For this review, take the finished solid that the model builds, in its own axes (mm). A direction names the side the tool comes from. Give positions to 0.01 mm unless a question says otherwise; leave off trailing zeros. Loops run counter-clockwise (first coordinate to the right, second up) from the corner with the lowest first, then second, coordinate; pieces in that order, holes last. Notation, with made-up numbers: (6, -37.5) -> (10, -37.5) arc R32 ccw to (10, -5.5) -> close; hole circle Ø10 at (33.5, -11). An arc over 180 degrees is marked (long way). One line per question, with ' | ' between items. Start each with the question number.
(1) Consider section A-A (x = -10). Write out the cut boundary in (y, z).
(2) Consider section C-C (x = 63). Write out the cut boundary in (y, z).
(3) Tool access review of faces 4 (the cylindrical face through (26.393, -27.015, 1.521)), 5 (the cylindrical face through (-61.468, -83.668, 1.479)): name each direction out of +Z, -Z, +X, -X, +Y, -Y from which nothing blocks a thin tool from reaching the whole face with its end or side.
(4) Draft analysis for pull direction Y (two halves, no side actions). For faces 1 (the cylindrical face through (-62.168, 39.968, 1.479)), 2 (the flat face through (1, -37, 0)), 3 (the cylindrical face through (38.289, -48.554, 1.521)), state which applies: +Y half, -Y half, draft (parallel to the pull), parting line (faces both ways), or undercut.
(5) Consider section D-D (z = 1.75). Give the number of separate pieces and of enclosed holes in the cut face, and give its area (3 significant figures).
(6) Consider section B-B (y = -64). Write out the cut boundary in (x, z).
(7) Wall thickness on probe 1 along Y at (x, z) = (-4.5, 0.95); probe 2 along Y at (x, z) = (-31, 1.05); probe 3 along Y at (x, z) = (-49, 1.45): over which ranges is each line inside the solid? List them lowest first.
(8) Insertion check: P1, Ø8, axis at x = 39.5, y = -64.5, coming from the -Z side; P2, Ø22, axis at x = -48.08, y = -71.5, coming from the -Z side; P3, Ø1.5, axis at y = -82, z = 2, coming from the -X side. Each pin has a flat end and moves straight along its axis. Give the tip position at first contact, or say it passes through.
from build123d import *

# Parameters (mm, degrees)
BOSS_EXTRUDE1_DEPTH = 3
SKETCH2_R           = 12.039123234
SKETCH2_R_2         = 12.323940374
SKETCH2_R_3         = 12.062522367
SKETCH2_R_4         = 17.95917031
SKETCH2_W           = 3
SKETCH2_H           = 18
SKETCH2_W_2         = 45
SKETCH2_H_2         = 1.6
SKETCH2_W_3         = 40
SKETCH2_H_3         = 3
CUT_EXTRUDE1_DEPTH  = 10


with BuildPart() as part:
    # Sketch1 → Boss-Extrude1 (new body)
    with BuildSketch(Plane.XY):
        with BuildLine():
            Line((-30, 53.5), (30, 53.5))
            ThreePointArc((30, 53.5), (61.819805153, 40.319805153), (75, 8.5))
            Line((75, 8.5), (75, -51.5))
            ThreePointArc((75, -51.5), (61.819805153, -83.319805153), (30, -96.5))
            Line((30, -96.5), (0.5, -96.5))
            Line((0.5, -96.5), (-0.5, -96.5))
            Line((-0.5, -96.5), (-30, -96.5))
            ThreePointArc((-30, -96.5), (-61.819805153, -83.319805153), (-75, -51.5))
            Line((-75, -51.5), (-75, 8.5))
            ThreePointArc((-75, 8.5), (-61.819805153, 40.319805153), (-30, 53.5))
        make_face()
    extrude(amount=BOSS_EXTRUDE1_DEPTH)

    # Sketch2 → Cut-Extrude1 (cut)
    with BuildSketch(Plane.XY.offset(3)):
        with Locations((-17.315529095, -57.691685277)):
            Circle(SKETCH2_R)
        with Locations((-48.082177359, -71.5)):
            Circle(SKETCH2_R_2)
        with Locations((48.082177359, -71.5)):
            Circle(SKETCH2_R_2)
        with Locations((17.315529095, -57.691685277)):
            Circle(SKETCH2_R)
        with Locations((-58.337726781, -5.217073599)):
            Circle(SKETCH2_R_3)
        with Locations((-52.54111189, -37.626479887)):
            Circle(SKETCH2_R_4)
        with Locations((52.54111189, -37.626479887)):
            Circle(SKETCH2_R_4)
        with Locations((58.337726781, -5.217073599)):
            Circle(SKETCH2_R_3)
        with Locations((-28.5, -80.5)):
            Rectangle(SKETCH2_W, SKETCH2_H)
        with Locations((28.5, -80.5)):
            Rectangle(SKETCH2_W, SKETCH2_H)
        with Locations((0, -13.3)):
            Rectangle(SKETCH2_W_2, SKETCH2_H_2)
        with Locations((0, -41.5)):
            Rectangle(SKETCH2_W_3, SKETCH2_H_3)
        with BuildLine():
            Line((-32, 44.093276202), (32, 44.093276202))
            ThreePointArc((32, 44.093276202), (54, 22.093276202), (32, 0.093276202))
            Line((32, 0.093276202), (-32, 0.093276202))
            ThreePointArc((-32, 0.093276202), (-54, 22.093276202), (-32, 44.093276202))
        make_face()
        with BuildLine():
            Line((-16.972534131, -17.799407518), (16.972534131, -17.799407518))
            ThreePointArc((16.972534131, -17.799407518), (26.395425928, -27.222299315), (16.972534131, -36.645191111))
            Line((16.972534131, -36.645191111), (-16.972534131, -36.645191111))
            ThreePointArc((-16.972534131, -36.645191111), (-26.395425928, -27.222299315), (-16.972534131, -17.799407518))
        make_face()
    extrude(amount=-CUT_EXTRUDE1_DEPTH, mode=Mode.SUBTRACT)


solid = part.part
A:
1) outline: (-96.5, 0) -> (-67.25, 0) -> (-67.25, 3) -> (-96.5, 3) -> close; (-48.13, 0) -> (-43, 0) -> (-43, 3) -> (-48.13, 3) -> close; (-40, 0) -> (-36.65, 0) -> (-36.65, 3) -> (-40, 3) -> close; (-17.8, 0) -> (-14.1, 0) -> (-14.1, 3) -> (-17.8, 3) -> close; (-12.5, 0) -> (0.09, 0) -> (0.09, 3) -> (-12.5, 3) -> close; (44.09, 0) -> (53.5, 0) -> (53.5, 3) -> (44.09, 3) -> close
2) outline: (-82.09, 0) -> (-52.23, 0) -> (-52.23, 3) -> (-82.09, 3) -> close; (-23.03, 0) -> (-16.34, 0) -> (-16.34, 3) -> (-23.03, 3) -> close; (5.91, 0) -> (39.09, 0) -> (39.09, 3) -> (5.91, 3) -> close
3) face 4: +Z, -Z | face 5: +Z, -Z, -X, -Y
4) face 1: +Y half | face 2: draft | face 3: undercut
5) separate pieces: 1 | enclosed holes: 14 | area: 10,400 mm^2
6) outline: (-73.23, 0) -> (-57.86, 0) -> (-57.86, 3) -> (-73.23, 3) -> close; (-38.3, 0) -> (-27.57, 0) -> (-27.57, 3) -> (-38.3, 3) -> close; (-7.06, 0) -> (7.06, 0) -> (7.06, 3) -> (-7.06, 3) -> close; (27.57, 0) -> (38.3, 0) -> (38.3, 3) -> (27.57, 3) -> close; (57.86, 0) -> (73.23, 0) -> (73.23, 3) -> (57.86, 3) -> close
7) probe 1: y = -96.5 to -43, -40 to -36.65, -17.8 to -14.1, -12.5 to 0.09, 44.09 to 53.5 | probe 2: y = -96.49 to 0.09, 44.09 to 53.49 | probe 3: y = -92.29 to -83.79, -59.21 to -55.23, -20.02 to -12.85, 2.42 to 8.13, 36.06 to 49.29
8) P1: stops at z = 0 | P2: passes through | P3: stops at x = -63.76
